For this review, take the finished solid that the model builds, in its own axes (mm). A direction names the side the tool comes from. Give positions to 0.01 mm unless a question says otherwise; leave off trailing zeros. Loops run counter-clockwise (first coordinate to the right, second up) from the corner with the lowest first, then second, coordinate; pieces in that order, holes last. Notation, with made-up numbers: (57, 5) - (85, 5) arc R35 ccw to (85, 39) - close; hole circle Ø2 at (65.25, 74.5). An arc over 180 degrees is marked (long way). Put each result on its own line as item: value.
from build123d import *

# Parameters (mm, degrees)
SKETCH1_W           = 22.0472
SKETCH1_H           = 36.322
BOSS_EXTRUDE1_DEPTH = 2.3876
CUT_EXTRUDE1_REACH  = 44.557
SKETCH2_R           = 1.7272
SKETCH2_R_2         = 8.89
SKETCH3_R           = 9.4615
BOSS_EXTRUDE2_DEPTH = 18.2626
CHAMFER1_SIZE       = 1.1303
CHAMFER1_SIZE2      = 0.158853305


with BuildPart() as part:
    # Sketch1 → Boss-Extrude1 (new body)
    with BuildSketch(Plane.XY):
        with Locations((11.0236, 18.161)):
            Rectangle(SKETCH1_W, SKETCH1_H)
    extrude(amount=BOSS_EXTRUDE1_DEPTH)

    # Sketch2 → Cut-Extrude1 (cut, up to next)
    with BuildSketch(Plane(origin=(0, 0, 0), x_dir=(-1, 0, 0), z_dir=(0, 0, -1)), mode=Mode.PRIVATE) as cut_extrude1_sk1:
        with Locations((-11.0236, 31.6484)):
            Circle(SKETCH2_R)
    cut_extrude1_tool1 = extrude(cut_extrude1_sk1.sketch, amount=-CUT_EXTRUDE1_REACH, mode=Mode.PRIVATE) & part.part
    # Sketch2 → Cut-Extrude1 (cut, up to next)
    with BuildSketch(Plane(origin=(0, 0, 0), x_dir=(-1, 0, 0), z_dir=(0, 0, -1)), mode=Mode.PRIVATE) as cut_extrude1_sk2:
        with Locations((-11.0236, 4.6736)):
            Circle(SKETCH2_R)
    cut_extrude1_tool2 = extrude(cut_extrude1_sk2.sketch, amount=-CUT_EXTRUDE1_REACH, mode=Mode.PRIVATE) & part.part
    # Sketch2 → Cut-Extrude1 (cut, up to next)
    with BuildSketch(Plane(origin=(0, 0, 0), x_dir=(-1, 0, 0), z_dir=(0, 0, -1)), mode=Mode.PRIVATE) as cut_extrude1_sk3:
        with Locations((-11.0236, 18.161)):
            Circle(SKETCH2_R_2)
    cut_extrude1_tool3 = extrude(cut_extrude1_sk3.sketch, amount=-CUT_EXTRUDE1_REACH, mode=Mode.PRIVATE) & part.part
    add(cut_extrude1_tool1.solids().sort_by_distance((11.0236, 31.6484, 0))[0], mode=Mode.SUBTRACT)
    add(cut_extrude1_tool2.solids().sort_by_distance((11.0236, 4.6736, 0))[0], mode=Mode.SUBTRACT)
    add(cut_extrude1_tool3.solids().sort_by_distance((11.0236, 18.161, 0))[0], mode=Mode.SUBTRACT)

    # Sketch3 → Boss-Extrude2 (add)
    with BuildSketch(Plane.XY.offset(2.3876)):
        with Locations(Location((11.0236, 18.161, 0), (0, 0, 180))):
            Circle(SKETCH3_R)
    extrude(amount=BOSS_EXTRUDE2_DEPTH)

    # Chamfer1
    chamfer1_edges = [part.edges().sort_by_distance(p)[0] for p in [
        (12.7508, 31.6484, 0),
        (12.7508, 4.6736, 0),
    ]]
    chamfer1_side = [part.faces().sort_by_distance(p)[0] for p in [
        (11.0236, 0.424896071, 0),
    ]]
    chamfer(chamfer1_edges, length=CHAMFER1_SIZE, length2=CHAMFER1_SIZE2, reference=chamfer1_side[0])


solid = part.part
1) Take a section at A-A on y = 20.5. State the section outline as (x, z) points, and give its area (3 significant figures).
Geometry check:
outline: (0, 0) - (2.45, 0) - (2.45, 2.39) - (19.6, 2.39) - (19.6, 0) - (22.05, 0) - (22.05, 2.39) - (20.19, 2.39) - (20.19, 20.65) - (1.86, 20.65) - (1.86, 2.39) - (0, 2.39) - close
area: 347 mm²
2) Take a section at B-B on x = 17. State the section outline as (y, z) points, and give its area (3 significant figures).
Geometry check:
outline: (0, 0) - (11.58, 0) - (11.58, 2.39) - (24.74, 2.39) - (24.74, 0) - (36.32, 0) - (36.32, 2.39) - (25.5, 2.39) - (25.5, 20.65) - (10.83, 20.65) - (10.83, 2.39) - (0, 2.39) - close
area: 323 mm²
3) Take a section at D-D on x = 11.75. State how many separate pieces and enclosed holes the cut face has, and give its area (3 significant figures).
Geometry check:
separate pieces: 3
enclosed holes: 0
area: 374 mm²
4) For faces 4 (the face through (11, 18, 2.388)), 5 (the face through (12.3, 5.84, 1.26)), 6 (the face through (6, 26.5, 2.388)), list the 3-axis set-ups (+Z, -Z, +X, -X, +Y, -Y) from which the entire face can be reached by the end or side of a thin tool; tool diameter is ignored.
Geometry check:
face 4: -Z
face 5: +Z, -Z
face 6: +Z
5) Insertion check: pin 1 Ø8 at (y, z) = (18.5, 15.5) entering from -X; pin 2 Ø8 at (y, z) = (24.5, 14.5) entering from -X; pin 3 Ø8 at (x, z) = (18, 9.5) entering from -Y. Each pin has a flat end and moves straight along its axis. Give the tip position at first contact, or say it passes through.
Geometry check:
pin 1: stops at x = 1.56
pin 2: stops at x = 1.86
pin 3: stops at y = 9.18
6) Wall thickness on line 1 (Z direction, x = 6, y = 2); line 2 (Y direction, x = 11.25, z = 2.5); line 3 (Y direction, x = 16.5, z = 10): over which ranges is each line inside the solid? List them lowest first.
Geometry check:
line 1: z = 0 to 2.39
line 2: y = 8.7 to 27.62
line 3: y = 10.45 to 25.88
7) Draft analysis for pull direction Y (two halves, no side actions). For faces 1 (the face through (11, 18, 20.65)), 2 (the face through (11, 0, 1)), 3 (the face through (12.297, 32.816, 1.258)), state which applies: pulls with the +Y half, pulls with the -Y half, needs draft (parallel to the pull), parting line crosses it, or undercut.
Geometry check:
face 1: needs draft
face 2: pulls with the -Y half
face 3: undercut
8) Take a section at C-C on z = 9.25. State the section outline as (x, y) points.
Geometry check:
outline: circle Ø18.92 at (11.02, 18.16)
